Design review of the part built by this model. Coordinates are the model's own, in mm. Face numbers are marked on the shaded views. Coordinates: 2 decimals unless noted, no trailing zeros. Write each loop counter-clockwise with the first axis right and the second up, starting at its lowest first coordinate (ties: lowest second). Pieces come first, ordered by that corner, then holes. Notation, with made-up numbers: (-3, 17.5) - (13, 17.5) arc R14 cw to (13, 21.5) - close; hole circle Ø5 at (-17, 0.25). An arc over 180 degrees is marked (long way). Answer as a JSON object with one key per item and string values.
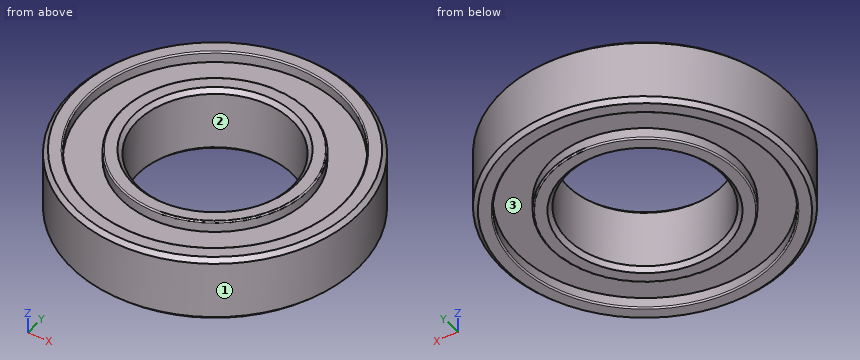
```python
from build123d import *

# Parameters (mm, degrees)
SKETCH_1_R          = 26
SKETCH_1_R_2        = 14
EXTRUDE_1_DEPTH     = 6
SKETCH_2_R          = 23
SKETCH_2_R_2        = 17
CUT_EXTRUDE_1_DEPTH = 2
CHAMFER_1_SIZE      = 0.75
FILLET_1_R          = 0.25


with BuildPart() as part:
    # 草图1 → 凸台-拉伸1 (new, symmetric)
    with BuildSketch(Plane.XY):
        Circle(SKETCH_1_R)
        Circle(SKETCH_1_R_2, mode=Mode.SUBTRACT)
    extrude(amount=EXTRUDE_1_DEPTH, both=True)

    # 草图2 → 切除-拉伸1 (cut)
    with BuildSketch(Plane.XY.offset(6)):
        Circle(SKETCH_2_R)
        Circle(SKETCH_2_R_2, mode=Mode.SUBTRACT)
    cut_extrude_1 = extrude(amount=-CUT_EXTRUDE_1_DEPTH, mode=Mode.SUBTRACT)

    # 镜向1: 切除-拉伸1 across plane
    add(cut_extrude_1.mirror(Plane.XY), mode=Mode.SUBTRACT)

    # 倒角1
    chamfer_1_edges = [part.edges().sort_by_distance(p)[0] for p in [
        (-26, 0, -6),
        (-26, 0, 6),
        (-14, 0, -6),
        (-14, 0, 6),
    ]]
    chamfer(chamfer_1_edges, length=CHAMFER_1_SIZE)

    # 圆角1
    fillet_1_edges = [part.edges().sort_by_distance(p)[0] for p in [
        (-17, 0, 6),
        (-23, 0, 6),
        (-23, 0, -6),
        (-17, 0, -6),
    ]]
    fillet(fillet_1_edges, radius=FILLET_1_R)


solid = part.part
```
(1) For pin 1 (3 mm diameter, centred on y = -10, z = -1.5, fed in from +X); pin 2 (5 mm diameter, centred on y = 19.5, z = -3.5, fed in from -X); pin 3 (1 mm diameter, centred on x = -14, z = 4, fed in from +Y); pin 4 (4 mm diameter, centred on x = 8.5, y = 19.5, fed in from +Z), all flat-tipped, find the tip position at first contact; note any pin that passes through.
Solved:
{"pin 1": "stops at x = 24.57", "pin 2": "stops at x = -19.67", "pin 3": "stops at y = 22.22", "pin 4": "stops at z = 6"}
(2) Take a section at A-A, the plane z = -0.5. Write out the cut boundary in (x, y), and give its area (3 significant figures).
Solved:
{"outline": "circle Ø52 at (0, 0); hole circle Ø28 at (0, 0)", "area": "1,510 mm^2"}
(3) The part is to be moulded in two halves that separate along Y. For the marked faces 1, 2 and 3, say which applies: pulls with the +Y half, pulls with the -Y half, needs draft (parallel to the pull), parting line crosses it, or undercut.
Solved:
{"face 1": "parting line crosses it", "face 2": "undercut", "face 3": "undercut"}
(4) To check wall thickness, follow line 1 (Y direction, x = 0, z = 4.45); line 2 (Y direction, x = 0, z = -2); line 3 (X direction, y = 7.5, z = 4.75). State the ranges of each line that lie inside material, in increasing order. Write a range as from..to.
Solved:
{"line 1": "y = -26..-23, -17..-14, 14..17, 23..26", "line 2": "y = -26..-14, 14..26", "line 3": "x = -24.89..-21.74, -15.26..-11.82, 11.82..15.26, 21.74..24.89"}
